from build123d import *

# Parameters (mm, degrees)
F0_W     = 1066.8
F0_H     = 426.72
F1_DEPTH = 792.48
F2_W     = 609.6
F2_H     = 609.6
F3_DEPTH = 304.8
F4_W     = 609.6
F4_H     = 121.92
F4_W_2   = 243.84
F4_H_2   = 229.870439
F4_H_3   = 252.629858
F5_DEPTH = 15.24
F6_W     = 121.92
F6_H     = 15.24
F6_R     = 15.24
F7_DEPTH = 25.908
F8_R     = 4.572


with BuildPart() as f1:
    # F0 (on Top) → F1 (new body)
    with BuildSketch(Plane.XY):
        with Locations((1.187092, -46.394789)):
            Rectangle(F0_W, F0_H)
    extrude(amount=F1_DEPTH)

    # F2 (on face) → F3 (cut)
    with BuildSketch(Plane.XZ.offset(259.754789)):
        with Locations((77.387092, 304.8)):
            Rectangle(F2_W, F2_H)
    extrude(amount=-F3_DEPTH, mode=Mode.SUBTRACT)

    # F4 (on face) → F5 (join)
    with BuildSketch(Plane.XZ.offset(259.754789)):
        with Locations((77.387092, 701.04)):
            Rectangle(F4_W, F4_H)
        with Locations((-379.812908, 700.366654)):
            Rectangle(F4_W_2, F4_H)
        with Locations((-379.812908, 493.991434)):
            Rectangle(F4_W_2, F4_H_2)
        with Locations((-379.812908, 184.462944)):
            Rectangle(F4_W_2, F4_H_3)
    extrude(amount=F5_DEPTH)

    # F6 (on face) → F7 (join)
    with BuildSketch(Plane.XZ.offset(259.754789)):
        with Locations((-379.812908, 738.466654)):
            Rectangle(F6_W, F6_H)
        with Locations((-379.812908, 586.066654)):
            Rectangle(F6_W, F6_H)
        with Locations((-379.812908, 287.917873)):
            Rectangle(F6_W, F6_H)
        with Locations((-105.492908, 731.52)):
            Circle(F6_R)
        with Locations((260.267092, 731.52)):
            Circle(F6_R)
    extrude(amount=F7_DEPTH)

    # F8
    f8_edges = [f1.edges().sort_by_distance(p)[0] for p in [
        (-120.732908, -285.662789, 731.52),
        (245.027092, -285.662789, 731.52),
    ]]
    fillet(f8_edges, radius=F8_R)


solid = f1.part
Geometry check sheet. Reference: the model listing, model coordinates, mm. A direction names the side the tool comes from. Coordinates: 2 decimals unless noted, no trailing zeros. Order: outer loops, then holes, each group sorted by start corner. A loop starts at its lowest first (then second) coordinate and runs counter-clockwise, first axis right, second up. Notation, with made-up numbers: (-20.75, -22) -> (16.25, -22) arc R25 ccw to (16.25, -4) -> close; hole circle Ø7 at (39, 56). An arc over 180 degrees is marked (long way). Use a Markdown table: item, result. Add a question column.
1. Cross-section at A-A (y = -75). Enter the section's corners in (x, z), and give its area (3 significant figures).
2. Cross-section at D-D (x = -158.5). Enter the section's corners in (y, z).
3. Material ranges on L1, parallel to X at y = -139, z = 496; L2, parallel to Y at x = 199.5, z = 66.5; L3, parallel to Z at x = 270, y = -167, recorded low to high.
4. Cross-section at B-B (x = -454.5). Enter the section's corners in (y, z), and give its area (3 significant figures).
5. Go/stop test with flat-tipped pins: pin 1 Ø3 at (x, y) = (-395, -279) entering from -Z; pin 2 Ø8.5 at (y, z) = (-279.5, 737) entering from -X; pin 3 Ø7.5 at (x, y) = (-373.5, -269.5) entering from +Z. Record where each tip stops, or that it passes through.
6. Mould release check, pull along Z, two halves, no side actions. Record for faces 4 (the face through (-6, -43, 792.48)), 5 (the face through (-382, -274.995, 701)), 6 (the face through (534.587, -49, 391)), 7 (the face through (-382, -274.995, 496)): pulls with the +Z half, pulls with the -Z half, needs draft (parallel to the pull), parting line crosses it, or undercut.
7. Cross-section at C-C (z = 528). Enter the section's corners in (x, y), and give its area (3 significant figures).
8. Set-up check for faces 1 (the face through (73, 45.045, 309)), 2 (the face through (-98.46, -278, 718)), 3 (the face through (-532.213, -49, 391)): record each of +Z, -Z, +X, -X, +Y, -Y from which the full face is reachable in a straight line by a thin tool's end or side.
Filled sheet:
| question | item | result |
|---|---|---|
| 1 | outline | (-532.21, 0) -> (-227.41, 0) -> (-227.41, 609.6) -> (382.19, 609.6) -> (382.19, 0) -> (534.59, 0) -> (534.59, 792.48) -> (-532.21, 792.48) -> close |
| 1 | area | 474,000 mm2 |
| 2 | outline | (-274.99, 640.08) -> (-259.75, 640.08) -> (-259.75, 609.6) -> (45.05, 609.6) -> (45.05, 0) -> (166.97, 0) -> (166.97, 792.48) -> (-259.75, 792.48) -> (-259.75, 762) -> (-274.99, 762) -> close |
| 3 | L1 | -532.21 to -227.41, 382.19 to 534.59 |
| 3 | L2 | 45.05 to 166.97 |
| 3 | L3 | 609.6 to 792.48 |
| 4 | outline | (-274.99, 58.15) -> (-259.75, 58.15) -> (-259.75, 0) -> (166.97, 0) -> (166.97, 792.48) -> (-259.75, 792.48) -> (-259.75, 761.33) -> (-274.99, 761.33) -> (-274.99, 639.41) -> (-259.75, 639.41) -> (-259.75, 608.93) -> (-274.99, 608.93) -> (-274.99, 379.06) -> (-259.75, 379.06) -> (-259.75, 310.78) -> (-274.99, 310.78) -> close |
| 4 | area | 347,000 mm2 |
| 5 | pin 1 | z = 280.3 |
| 5 | pin 2 | x = -440.77 |
| 5 | pin 3 | z = 761.33 |
| 6 | face 4 | pulls with the +Z half |
| 6 | face 5 | undercut |
| 6 | face 6 | needs draft |
| 6 | face 7 | undercut |
| 7 | outline | (-532.21, -259.75) -> (-501.73, -259.75) -> (-501.73, -274.99) -> (-257.89, -274.99) -> (-257.89, -259.75) -> (-227.41, -259.75) -> (-227.41, 45.05) -> (382.19, 45.05) -> (382.19, -259.75) -> (534.59, -259.75) -> (534.59, 166.97) -> (-532.21, 166.97) -> close |
| 7 | area | 273,000 mm2 |
| 8 | face 1 | -Z, -Y |
| 8 | face 2 | -Y |
| 8 | face 3 | +Z, -Z, -X, +Y, -Y |
